For this review, use the dimensioned drawing (mm, ordinates from the lowest corner) and the shaded views. A direction names the side the tool comes from. Round coordinates to 2 decimals unless told otherwise and drop trailing zeros. Write each loop counter-clockwise with the first axis right and the second up, starting at its lowest first coordinate (ties: lowest second). Pieces come first, ordered by that corner, then holes. Notation, with made-up numbers: M 42,38 L 93,38 A6 cw 93,45 Z; hole C 26.5,57 d4. An arc over 180 degrees is marked long. One line per question, with ' | ' between items. Start each with the question number.
Item 1: Add section A-A, the plane y = 5. State the section outline as (x, z) points.
Item 2: Add section B-B, the plane z = 19. State the section outline as (x, y) points.
Item 3: Machinability: for the marked faces 1 and 2, which of the approach directions +Z, -Z, +X, -X, +Y, -Y give a long, thin tool a straight path to every point of the face, cutting with its end or side? Answer none if there is none.
Item 4: For L1, parallel to X at y = 36.5, z = 5; L2, parallel to Y at x = 12, z = 18, list the stretches that pass through material, from the lowest coordinate up.
Item 5: Add section C-C, the plane x = 55. State the section outline as (y, z) points.
Item 6: Insertion check: pin 1 Ø8 at (y, z) = (12.5, 23.5) entering from +X; pin 2 Ø16.5 at (x, z) = (25, 17) entering from +Y. Each pin has a flat end and moves straight along its axis. Give the tip position at first contact, or say it passes through.
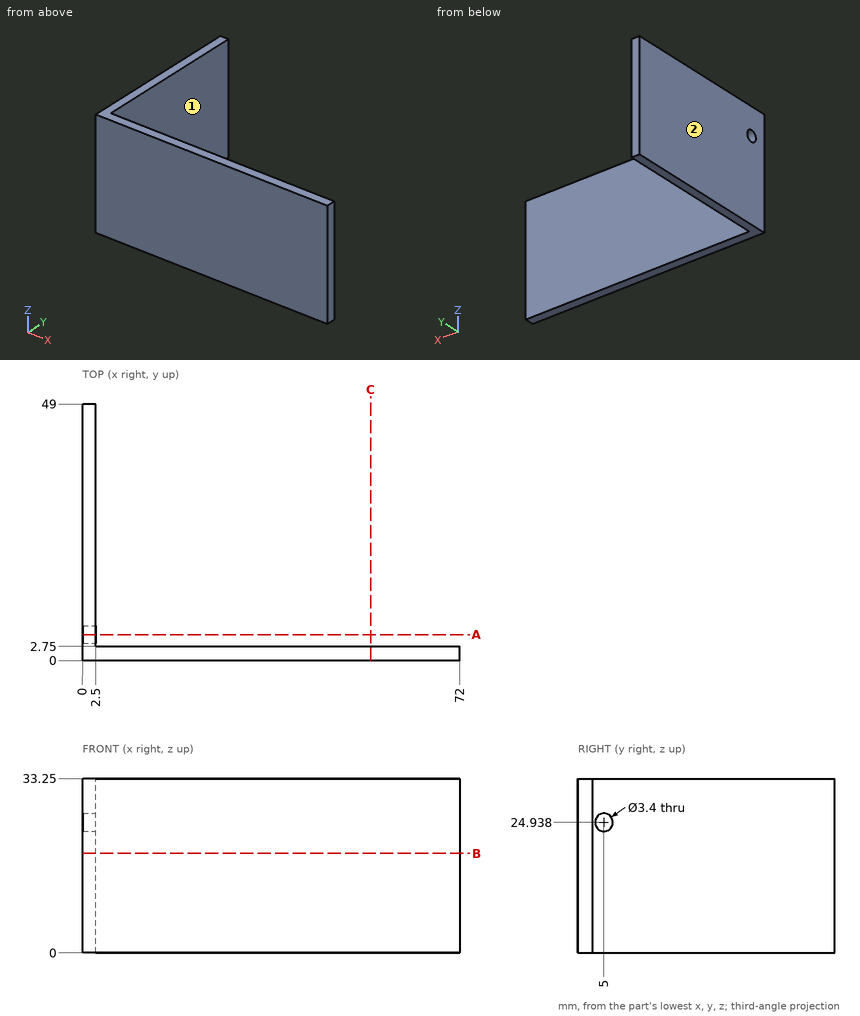
Computed values:
1) outline: M 0,0 L 2.5,0 L 2.5,23.24 L 0,23.24 Z; M 0,26.64 L 2.5,26.64 L 2.5,33.25 L 0,33.25 Z
2) outline: M 0,0 L 72,0 L 72,2.75 L 2.5,2.75 L 2.5,49 L 0,49 Z
3) face 1: +Z, -Z, +X, +Y | face 2: +Z, -Z, -X, +Y, -Y
4) L1: x = 0 to 2.5 | L2: y = 0 to 2.75
5) outline: M 0,0 L 2.75,0 L 2.75,33.25 L 0,33.25 Z
6) pin 1: stops at x = 2.5 | pin 2: stops at y = 2.75
